Read the model definition and answer for the solid it produces. Units are mm, in the model's axes. Face numbers are marked on the shaded views. Coordinates: 2 decimals unless noted, no trailing zeros. Order: outer loops, then holes, each group sorted by start corner. A loop starts at its lowest first (then second) coordinate and runs counter-clockwise, first axis right, second up. Notation, with made-up numbers: M 11,52.5 L 44,52.5 A26 ccw 44,73.5 Z; hole C -15.75,44.25 d11. An arc over 180 degrees is marked long. Put each result on its own line as item: value.
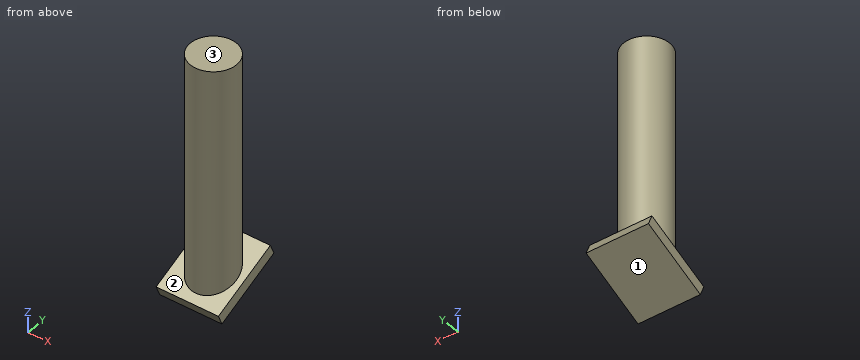
from build123d import *

# Parameters (mm, degrees)
F0_R     = 10
F1_DEPTH = 100
F3_DEPTH = 25
F4_W     = 27
F4_H     = 32
F5_DEPTH = 5


with BuildPart() as f1:
    # F0 (on Top) → F1 (new body)
    with BuildSketch(Plane.XY):
        with Locations((-12.7463750541, 13.7874316424)):
            Circle(F0_R)
    extrude(amount=F1_DEPTH)

    # F2 (on Right) → F3 (cut)
    with BuildSketch(Plane.YZ):
        Polygon((35.4767926037, 15.3907770291), (0, 0), (35.4767926037, 0), align=None)
    extrude(amount=-F3_DEPTH, mode=Mode.SUBTRACT)

    # F4 (on face) → F5 (join)
    with BuildSketch(Plane(origin=(0, 0, 0), x_dir=(1, 0, 0), z_dir=(0, 0.3979883977, -0.9173904487))):
        with Locations((-13.5, -16)):
            Rectangle(F4_W, F4_H)
    extrude(amount=F5_DEPTH)


solid = f1.part
Q1. Given pin 1 (8 mm diameter, centred on x = -24, z = 63.5, fed in from +Y); pin 2 (8 mm diameter, centred on x = -6, y = 8, fed in from -Z); pin 3 (4 mm diameter, centred on x = -18.5, y = 23.5, fed in from +Z); pin 4 (6 mm diameter, centred on y = 28, z = 51.5, fed in from -X), each flat-ended and moving along its own axis, determine where each tip first touches the part or whether it passes through.
Answers below:
pin 1: stops at y = 20.67
pin 2: stops at z = -3.71
pin 3: stops at z = 100
pin 4: passes through
Q2. Consider line 1 along Y through (x, z) = (-13, 63); line 2 along Z through (x, y) = (-15.5, 8.5); line 3 along Y through (x, z) = (-8.75, 81.5). Determine where each line is inside the solid, lowest interval first.
Answers below:
line 1: y = 3.79 to 23.78
line 2: z = -1.76 to 100
line 3: y = 4.62 to 22.95
Q3. Find section B-B on y = 6.5. Write down the section's boundary in (x, z), plus the area to 3 significant figures.
Answers below:
outline: M -27,-2.63 L 0,-2.63 L 0,2.82 L -5.9,2.82 L -5.9,100 L -19.59,100 L -19.59,2.82 L -27,2.82 Z
area: 1,480 mm^2
Q4. For a pull along Y with two mould halves and no side action, classify the marked faces 1, 2 and 3 as +Y half, -Y half, draft (parallel to the pull), parting line (faces both ways), or undercut.
Answers below:
face 1: +Y half
face 2: undercut
face 3: draft
Q5. Find section D-D on x = -14.75. Write down the section's boundary in (y, z).
Answers below:
outline: M 0,0 L 1.99,-4.59 L 31.35,8.15 L 29.36,12.74 L 23.58,10.23 L 23.58,100 L 3.99,100 L 3.99,1.73 Z
Q6. Find section C-C on z = 78. Write down the section's boundary in (x, y), plus the area to 3 significant figures.
Answers below:
outline: C -12.75,13.79 d20
area: 314 mm^2
Q7. Find section A-A on x = -24.5. Write down the section's boundary in (y, z).
Answers below:
outline: M 0,0 L 1.99,-4.59 L 31.35,8.15 L 29.36,12.74 Z
